from build123d import *

# Parameters (mm, degrees)
F0_W     = 37.1348839253
F0_H     = 12.7599176485
F1_DEPTH = 2.54
F2_W     = 4.0106745437
F2_H     = 1.6526868567
F3_DEPTH = 3.81
F4_W     = 5.08
F4_H     = 1.6526868567
F4_W_2   = 1.27
F4_W_3   = 2.7406745437
F4_W_4   = 2.3393254563
F4_H_2   = 2.54
F5_DEPTH = 3.81


with BuildPart() as f1:
    # F0 (on Top) → F1 (new body)
    with BuildSketch(Plane.XY):
        with Locations((-0.831102021, -8.5664497456)):
            Rectangle(F0_W, F0_H)
    extrude(amount=F1_DEPTH)

    # F2 (on face) → F3 (join)
    with BuildSketch(Plane.XY.offset(2.54)):
        with Locations((-0.302497996, -7.8425793909)):
            Rectangle(F2_W, F2_H)
    extrude(amount=F3_DEPTH)

    # F4 (on face) → F5 (join)
    with BuildSketch(Plane.XY.offset(6.35)):
        with Locations((-4.8478352679, -7.8425793909)):
            Rectangle(F4_W, F4_H)
        with Locations((-1.6728352679, -7.8425793909)):
            Rectangle(F4_W_2, F4_H)
        with Locations((0.332502004, -7.8425793909)):
            Rectangle(F4_W_3, F4_H)
        with Locations((2.872502004, -7.8425793909)):
            Rectangle(F4_W_4, F4_H)
        with Locations((-1.6728352679, -5.7462359625)):
            Rectangle(F4_W_2, F4_H_2)
        with Locations((-1.6728352679, -9.9389228192)):
            Rectangle(F4_W_2, F4_H_2)
    extrude(amount=F5_DEPTH)


solid = f1.part
Read the model definition and answer for the solid it produces. Units are mm, in the model's axes. A direction names the side the tool comes from. Give positions to 0.01 mm unless a question says otherwise; leave off trailing zeros. Write each loop counter-clockwise with the first axis right and the second up, starting at its lowest first coordinate (ties: lowest second). Pieces come first, ordered by that corner, then holes. Notation, with made-up numbers: (32, 26) - (77, 26) arc R10 ccw to (77, 36) - close; hole circle Ø7 at (-3, 70). An arc over 180 degrees is marked (long way). Use CSV: the item, a comma, the result in double quotes. Start each with the question number.
(1) Consider line 1 along Z through (x, y) = (4, -10.25); line 2 along Y through (x, z) = (-3.5, 8); line 3 along Z through (x, y) = (-2.5, -8). Determine where each line is inside the solid, lowest interval first.
(2) For faces 1 (the flat face through (4.042, -8, 8)), 2 (the flat face through (-2, -10, 6.35)), 3 (the flat face through (-5, -7.016, 8)), 4 (the flat face through (-1.038, -10, 8)), 5 (the flat face through (1.703, -8, 4)), determine the directions among +Z, -Z, +X, -X, +Y, -Y from which every point of the face is accessible in a straight line to the end or side of a thin tool.
(3) Find section D-D (x = -1.5). Give the vertices of the cut face in (y, z).
(4) Find section A-A (x = 3). Give the vertices of the cut face in (y, z), plus the area to 3 significant figures.
(5) Find section B-B (y = -9.5). Give the vertices of the cut face in (x, z), plus the area to 3 significant figures.
(6) Determine the mould class of faces 6 (the flat face through (-2, -8, 10.16)), 7 (the flat face through (1, -8.669, 6)), 8 (the flat face through (-2, -11.209, 8)) for opening direction Z: +Z half, -Z half, draft (parallel to the pull), parting line (faces both ways), or undercut.
(7) Given P1, Ø0.8, axis at y = -10, z = 8, coming from the -X side; P2, Ø6, axis at y = -6.5, z = 7, coming from the +X side; P3, Ø1.1, axis at x = -5.5, z = 8.5, coming from the -Y side; P4, Ø5, axis at x = 2.5, z = 4.5, coming from the -Y side, each flat-ended and moving along its own axis, determine where each tip first touches the part or whether it passes through.
(8) Find section C-C (z = 8). Give the vertices of the cut face in (x, y), plus the area to 3 significant figures.
Findings below:
1,line 1,"0 to 2.54"
1,line 2,"-8.67 to -7.02"
1,line 3,"0 to 2.54, 6.35 to 10.16"
2,face 1,"+Z, +X, +Y, -Y"
2,face 2,"+X, -X, -Y"
2,face 3,"+Z, -X, +Y"
2,face 4,"+Z, +X, -Y"
2,face 5,"+X, +Y, -Y"
3,outline,"(-14.95, 0) - (-2.19, 0) - (-2.19, 2.54) - (-7.02, 2.54) - (-7.02, 6.35) - (-4.48, 6.35) - (-4.48, 10.16) - (-11.21, 10.16) - (-11.21, 6.35) - (-8.67, 6.35) - (-8.67, 2.54) - (-14.95, 2.54) - close"
4,outline,"(-14.95, 0) - (-2.19, 0) - (-2.19, 2.54) - (-14.95, 2.54) - close; (-8.67, 6.35) - (-7.02, 6.35) - (-7.02, 10.16) - (-8.67, 10.16) - close"
4,area,"38.7 mm2"
5,outline,"(-19.4, 0) - (17.74, 0) - (17.74, 2.54) - (-19.4, 2.54) - close; (-2.31, 6.35) - (-1.04, 6.35) - (-1.04, 10.16) - (-2.31, 10.16) - close"
5,area,"99.2 mm2"
6,face 6,"+Z half"
6,face 7,"undercut"
6,face 8,"draft"
7,P1,"x = -2.31"
7,P2,"x = 4.04"
7,P3,"y = -8.67"
7,P4,"y = -14.95"
8,outline,"(-7.39, -8.67) - (-2.31, -8.67) - (-2.31, -11.21) - (-1.04, -11.21) - (-1.04, -8.67) - (4.04, -8.67) - (4.04, -7.02) - (-1.04, -7.02) - (-1.04, -4.48) - (-2.31, -4.48) - (-2.31, -7.02) - (-7.39, -7.02) - close"
8,area,"25.3 mm2"
